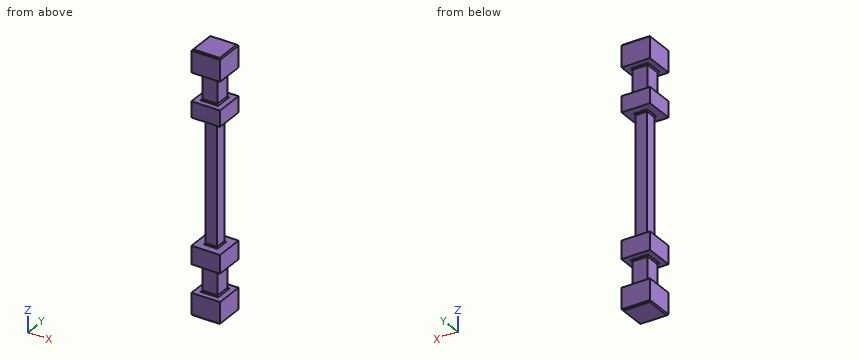
from build123d import *

# Parameters (mm, degrees)
F0_W      = 3.2004
F0_H      = 3.2004
F1_DEPTH  = 2.4892
F2_W      = 1.7018
F2_H      = 1.7018
F3_DEPTH  = 3.0988
F4_W      = 3.2004
F4_H      = 3.2004
F4_W_2    = 1.7018
F4_H_2    = 1.7018
F5_DEPTH  = 2.032
F6_W      = 1.27
F6_H      = 1.27
F7_DEPTH  = 13.97
F8_W      = 3.2004
F8_H      = 3.2004
F8_W_2    = 1.27
F8_H_2    = 1.27
F9_DEPTH  = 1.778
F10_W     = 1.7018
F10_H     = 1.7018
F11_DEPTH = 3.1242
F12_W     = 3.2004
F12_H     = 3.2004
F12_W_2   = 1.7018
F12_H_2   = 1.7018
F13_DEPTH = 2.5146
F14_SIZE2 = 0.127
F14_SIZE  = 0.127


with BuildPart() as f1:
    # F0 (on Top) → F1 (new body)
    with BuildSketch(Plane.XY):
        with Locations((1.6002, 1.6002)):
            Rectangle(F0_W, F0_H)
    extrude(amount=F1_DEPTH)

    # F2 (on face) → F3 (join)
    with BuildSketch(Plane.XY.offset(2.4892)):
        with Locations((1.6002, 1.6002)):
            Rectangle(F2_W, F2_H)
    extrude(amount=F3_DEPTH)

    # F4 (on face) → F5 (join)
    with BuildSketch(Plane.XY.offset(5.588)):
        with Locations((1.6002, 1.6002)):
            Rectangle(F4_W, F4_H)
        with Locations((1.6002, 1.6002)):
            Rectangle(F4_W_2, F4_H_2, mode=Mode.SUBTRACT)
        with Locations((1.6002, 1.6002)):
            Rectangle(F4_W_2, F4_H_2)
    extrude(amount=F5_DEPTH)

    # F6 (on face) → F7 (join)
    with BuildSketch(Plane.XY.offset(7.62)):
        with Locations((1.6002, 1.6002)):
            Rectangle(F6_W, F6_H)
    extrude(amount=F7_DEPTH)

    # F8 (on face) → F9 (join)
    with BuildSketch(Plane.XY.offset(21.59)):
        with Locations((1.6002, 1.6002)):
            Rectangle(F8_W, F8_H)
        with Locations((1.6002, 1.6002)):
            Rectangle(F8_W_2, F8_H_2, mode=Mode.SUBTRACT)
        with Locations((1.6002, 1.6002)):
            Rectangle(F8_W_2, F8_H_2)
    extrude(amount=F9_DEPTH)

    # F10 (on face) → F11 (join)
    with BuildSketch(Plane.XY.offset(23.368)):
        with Locations((1.6002, 1.6002)):
            Rectangle(F10_W, F10_H)
    extrude(amount=F11_DEPTH)

    # F12 (on face) → F13 (join)
    with BuildSketch(Plane.XY.offset(26.4922)):
        with Locations((1.6002, 1.6002)):
            Rectangle(F12_W, F12_H)
        with Locations((1.6002, 1.6002)):
            Rectangle(F12_W_2, F12_H_2, mode=Mode.SUBTRACT)
        with Locations((1.6002, 1.6002)):
            Rectangle(F12_W_2, F12_H_2)
    extrude(amount=F13_DEPTH)

    # F14
    f14_edges = [f1.edges().sort_by_distance(p)[0] for p in [
        (0.7493, 1.6002, 23.368),
        (1.6002, 0.7493, 23.368),
        (0, 1.6002, 29.0068),
        (1.6002, 3.2004, 29.0068),
        (3.2004, 1.6002, 29.0068),
        (1.6002, 0, 29.0068),
        (0.9652, 1.6002, 7.62),
        (1.6002, 0.9652, 7.62),
        (0.7493, 1.6002, 2.4892),
        (1.6002, 0.7493, 2.4892),
        (0, 1.6002, 0),
        (1.6002, 0, 0),
        (0.7493, 1.6002, 26.4922),
        (1.6002, 0.7493, 26.4922),
        (0.9652, 1.6002, 21.59),
        (1.6002, 0.9652, 21.59),
        (0.7493, 1.6002, 5.588),
        (1.6002, 0.7493, 5.588),
        (3.2004, 1.6002, 0),
        (1.6002, 3.2004, 0),
        (2.4511, 1.6002, 26.4922),
        (1.6002, 2.4511, 26.4922),
        (2.2352, 1.6002, 21.59),
        (1.6002, 2.2352, 21.59),
        (2.4511, 1.6002, 5.588),
        (1.6002, 2.4511, 5.588),
        (2.4511, 1.6002, 23.368),
        (1.6002, 2.4511, 23.368),
        (2.2352, 1.6002, 7.62),
        (1.6002, 2.2352, 7.62),
        (2.4511, 1.6002, 2.4892),
        (1.6002, 2.4511, 2.4892),
    ]]
    chamfer(f14_edges, length=F14_SIZE, length2=F14_SIZE2)


solid = f1.part
Design review of the part built by this model. Coordinates are the model's own, in mm. Give positions to 0.01 mm unless a question says otherwise; leave off trailing zeros. Write each loop counter-clockwise with the first axis right and the second up, starting at its lowest first coordinate (ties: lowest second). Pieces come first, ordered by that corner, then holes. Notation, with made-up numbers: M -37,43 L -19,43 A30 ccw -19,72 Z; hole C 46,82 d10. An arc over 180 degrees is marked long. Answer as a JSON object with one key per item and string values. Group by question number.
1) We need section B-B (z = 15.75). Give the boundary of the cut face in (x, y), and give its area (3 significant figures).
2) Clearance check with flat-ended pins moving along their axes: pin 1 Ø1.4 at (y, z) = (2, 4) entering from -X; pin 2 Ø0.9 at (y, z) = (1.5, 25.5) entering from +X; pin 3 Ø1 at (x, z) = (1.5, 20) entering from -Y. State where each tip first meets the part, or that it passes through.
3) We need section A-A (z = 4). Give the boundary of the cut face in (x, y).
4) For line 1 along Z through (x, y) = (2.1, 3); line 2 along Y through (x, z) = (1.9, 4); line 3 along Y through (x, z) = (1.5, 14.5), list the stretches that pass through material, from the lowest coordinate up.
Answer key:
{
 "1": {"outline": "M 0.97,0.97 L 2.24,0.97 L 2.24,2.24 L 0.97,2.24 Z", "area": "1.61 mm²"},
 "2": {"pin 1": "stops at x = 0.75", "pin 2": "stops at x = 2.45", "pin 3": "stops at y = 0.97"},
 "3": {"outline": "M 0.75,0.75 L 2.45,0.75 L 2.45,2.45 L 0.75,2.45 Z"},
 "4": {"line 1": "z = 0 to 2.49, 5.59 to 7.62, 21.59 to 23.37, 26.49 to 29.01", "line 2": "y = 0.75 to 2.45", "line 3": "y = 0.97 to 2.24"}
}
